Can you work these out from the model? Positions are in its coordinate system, mm. A direction names the side the tool comes from. Coordinates: 2 decimals unless noted, no trailing zeros. Order: outer loops, then holes, each group sorted by start corner. A loop starts at its lowest first (then second) coordinate and runs counter-clockwise, first axis right, second up. Notation, with made-up numbers: (-6, 50) -> (1, 50) arc R14 cw to (1, 56) -> close; hole circle Ø6 at (11, 30). An arc over 180 degrees is marked (long way). Answer as CSV lines item,"result".
from build123d import *

# Parameters (mm, degrees)
SKETCH1_W           = 240
SKETCH1_H           = 65
BOSS_EXTRUDE1_DEPTH = 3
SKETCH2_W           = 6
SKETCH2_H           = 16
SKETCH2_W_2         = 65
SKETCH2_H_2         = 8
CUT_EXTRUDE1_DEPTH  = 6
SKETCH3_W           = 20
SKETCH3_H           = 6
CUT_EXTRUDE2_DEPTH  = 6


with BuildPart() as part:
    # Sketch1 → Boss-Extrude1 (new body, symmetric)
    with BuildSketch(Plane.XY):
        Rectangle(SKETCH1_W, SKETCH1_H)
    extrude(amount=BOSS_EXTRUDE1_DEPTH, both=True)

    # Sketch2 → Cut-Extrude1 (cut)
    with BuildSketch(Plane.XY.offset(3)):
        with Locations((-117, -24.5)):
            Rectangle(SKETCH2_W, SKETCH2_H)
        with Locations((-57.5, -28.5)):
            Rectangle(SKETCH2_W_2, SKETCH2_H_2)
        with Locations((57.5, -28.5)):
            Rectangle(SKETCH2_W_2, SKETCH2_H_2)
        with Locations((117, -24.5)):
            Rectangle(SKETCH2_W, SKETCH2_H)
    extrude(amount=-CUT_EXTRUDE1_DEPTH, mode=Mode.SUBTRACT)

    # Sketch3 → Cut-Extrude2 (cut)
    with BuildSketch(Plane.XY.offset(3)):
        with Locations((-80, 29.5)):
            Rectangle(SKETCH3_W, SKETCH3_H)
        with Locations((-40, 29.5)):
            Rectangle(SKETCH3_W, SKETCH3_H)
        with Locations((0, 29.5)):
            Rectangle(SKETCH3_W, SKETCH3_H)
        with Locations((40, 29.5)):
            Rectangle(SKETCH3_W, SKETCH3_H)
        with Locations((80, 29.5)):
            Rectangle(SKETCH3_W, SKETCH3_H)
    extrude(amount=-CUT_EXTRUDE2_DEPTH, mode=Mode.SUBTRACT)


solid = part.part
Q1. If I drill on line 1 (X direction, y = -26, z = -0.5); line 2 (X direction, y = 29.5, z = -0.2); line 3 (X direction, y = -18, z = 1.4), over which ranges is the centre line in solid material (lowest first)?
Solution:
line 1,"-114 to -90, -25 to 25, 90 to 114"
line 2,"-120 to -90, -70 to -50, -30 to -10, 10 to 30, 50 to 70, 90 to 120"
line 3,"-114 to 114"
Q2. Which directions (+Z, -Z, +X, -X, +Y, -Y) give clear straight access to the entire face, cutting with the end or side of a thin tool? Please do faces 1 (the flat face through (-117, -16.5, 0)), 2 (the flat face through (-25, -29, 0)), 3 (the flat face through (-90, 29, 0)), 4 (the flat face through (20, 32.5, 0)).
Solution:
face 1,"+Z, -Z, -X, -Y"
face 2,"+Z, -Z, -Y"
face 3,"+Z, -Z, +Y"
face 4,"+Z, -Z, +X, -X, +Y"
Q3. Imagine slicing it at A-A (x = 8). List the corners of the cut face in (y, z) for me.
Solution:
outline,"(-32.5, -3) -> (26.5, -3) -> (26.5, 3) -> (-32.5, 3) -> close"
Q4. Imagine slicing it at B-B (y = -20.5). List the corners of the cut face in (x, z) for me.
Solution:
outline,"(-114, -3) -> (114, -3) -> (114, 3) -> (-114, 3) -> close"
Q5. For P1, Ø3, axis at y = -28.5, z = 0.5, coming from the -X side; P2, Ø1.8, axis at x = -2, z = 1, coming from the +Y side; P3, Ø1.8, axis at x = -118, z = -1.5, coming from the -Y side, each with a flat end and sliding along its axis, tell me the tip position at first contact or that it passes through.
Solution:
P1,"x = -114"
P2,"y = 26.5"
P3,"y = -16.5"
